Verification items for the finished model (mm, model axes). A direction names the side the tool comes from. Give positions to 0.01 mm unless a question says otherwise; leave off trailing zeros. Answer in a Markdown table with one row per item.
```python
from build123d import *

# Parameters (mm, degrees)
SKETCH1_R           = 13
BOSS_EXTRUDE1_DEPTH = 2
CUT_EXTRUDE1_DEPTH  = 2
CUT_EXTRUDE2_DEPTH  = 2


with BuildPart() as part:
    # Sketch1 → Boss-Extrude1 (new body)
    with BuildSketch(Plane.XY):
        Circle(SKETCH1_R)
    extrude(amount=BOSS_EXTRUDE1_DEPTH)

    # Sketch2 → Cut-Extrude1 (cut)
    with BuildSketch(Plane.XY.offset(2)):
        with BuildLine():
            Line((1.85, 2.101784956), (1.85, -2.101784956))
            ThreePointArc((1.85, -2.101784956), (0, -2.8), (-1.85, -2.101784956))
            Line((-1.85, -2.101784956), (-1.85, 2.101784956))
            ThreePointArc((-1.85, 2.101784956), (0, 2.8), (1.85, 2.101784956))
        make_face()
    extrude(amount=-CUT_EXTRUDE1_DEPTH, mode=Mode.SUBTRACT)

    # Sketch3 → Cut-Extrude2 (cut)
    with BuildSketch(Plane.XY.offset(2)):
        with BuildLine():
            Line((-0.421898485, 5.3), (0.421898485, 5.3))
            Line((0.421898485, 5.3), (1.025755042, 11.638206547))
            add(Edge.make_bspline(
                [(-1.025755042, 11.638206547), (0, 12.476130474), (1.025755042, 11.638206547)],
                knots=[0, 0, 0, 1, 1, 1], degree=2))
            Line((-1.025755042, 11.638206547), (-0.421898485, 5.3))
        make_face()
        with BuildLine():
            Line((2.039039374, 4.910225735), (4.571954624, 10.751616435))
            add(Edge.make_bspline(
                [(2.62085259, 11.385567915), (3.85533634, 11.865505185), (4.571954624, 10.751616435)],
                knots=[0, 0, 0, 1, 1, 1], degree=2))
            Line((2.62085259, 11.385567915), (1.236540767, 5.170973338))
            Line((1.236540767, 5.170973338), (2.039039374, 4.910225735))
        make_face()
        with BuildLine():
            Line((3.456584881, 4.039804363), (7.670619433, 8.812583195))
            add(Edge.make_bspline(
                [(6.01091291, 10.018430567), (7.333285498, 10.093401577), (7.670619433, 8.812583195)],
                knots=[0, 0, 0, 1, 1, 1], degree=2))
            Line((6.01091291, 10.018430567), (2.773938793, 4.535775778))
            Line((2.773938793, 4.535775778), (3.456584881, 4.039804363))
        make_face()
        with BuildLine():
            Line((4.535775778, 2.773938793), (10.018430567, 6.01091291))
            add(Edge.make_bspline(
                [(8.812583195, 7.670619433), (10.093401577, 7.333285498), (10.018430567, 6.01091291)],
                knots=[0, 0, 0, 1, 1, 1], degree=2))
            Line((8.812583195, 7.670619433), (4.039804363, 3.456584881))
            Line((4.039804363, 3.456584881), (4.535775778, 2.773938793))
        make_face()
        with BuildLine():
            Line((5.170973338, 1.236540767), (11.385567915, 2.62085259))
            add(Edge.make_bspline(
                [(10.751616435, 4.571954624), (11.865505185, 3.85533634), (11.385567915, 2.62085259)],
                knots=[0, 0, 0, 1, 1, 1], degree=2))
            Line((10.751616435, 4.571954624), (4.910225735, 2.039039374))
            Line((4.910225735, 2.039039374), (5.170973338, 1.236540767))
        make_face()
        with BuildLine():
            Line((5.3, -0.421898485), (11.638206547, -1.025755042))
            add(Edge.make_bspline(
                [(11.638206547, 1.025755042), (12.476130474, 0), (11.638206547, -1.025755042)],
                knots=[0, 0, 0, 1, 1, 1], degree=2))
            Line((11.638206547, 1.025755042), (5.3, 0.421898485))
            Line((5.3, 0.421898485), (5.3, -0.421898485))
        make_face()
        with BuildLine():
            Line((4.910225735, -2.039039374), (10.751616435, -4.571954624))
            add(Edge.make_bspline(
                [(11.385567915, -2.62085259), (11.865505185, -3.85533634), (10.751616435, -4.571954624)],
                knots=[0, 0, 0, 1, 1, 1], degree=2))
            Line((11.385567915, -2.62085259), (5.170973338, -1.236540767))
            Line((5.170973338, -1.236540767), (4.910225735, -2.039039374))
        make_face()
        with BuildLine():
            Line((4.039804363, -3.456584881), (8.812583195, -7.670619433))
            add(Edge.make_bspline(
                [(10.018430567, -6.01091291), (10.093401577, -7.333285498), (8.812583195, -7.670619433)],
                knots=[0, 0, 0, 1, 1, 1], degree=2))
            Line((10.018430567, -6.01091291), (4.535775778, -2.773938793))
            Line((4.535775778, -2.773938793), (4.039804363, -3.456584881))
        make_face()
        with BuildLine():
            Line((2.773938793, -4.535775778), (6.01091291, -10.018430567))
            add(Edge.make_bspline(
                [(7.670619433, -8.812583195), (7.333285498, -10.093401577), (6.01091291, -10.018430567)],
                knots=[0, 0, 0, 1, 1, 1], degree=2))
            Line((7.670619433, -8.812583195), (3.456584881, -4.039804363))
            Line((3.456584881, -4.039804363), (2.773938793, -4.535775778))
        make_face()
        with BuildLine():
            Line((1.236540767, -5.170973338), (2.62085259, -11.385567915))
            add(Edge.make_bspline(
                [(4.571954624, -10.751616435), (3.85533634, -11.865505185), (2.62085259, -11.385567915)],
                knots=[0, 0, 0, 1, 1, 1], degree=2))
            Line((4.571954624, -10.751616435), (2.039039374, -4.910225735))
            Line((2.039039374, -4.910225735), (1.236540767, -5.170973338))
        make_face()
        with BuildLine():
            Line((-0.421898485, -5.3), (-1.025755042, -11.638206547))
            add(Edge.make_bspline(
                [(1.025755042, -11.638206547), (0, -12.476130474), (-1.025755042, -11.638206547)],
                knots=[0, 0, 0, 1, 1, 1], degree=2))
            Line((1.025755042, -11.638206547), (0.421898485, -5.3))
            Line((0.421898485, -5.3), (-0.421898485, -5.3))
        make_face()
        with BuildLine():
            Line((-2.039039374, -4.910225735), (-4.571954624, -10.751616435))
            add(Edge.make_bspline(
                [(-2.62085259, -11.385567915), (-3.85533634, -11.865505185), (-4.571954624, -10.751616435)],
                knots=[0, 0, 0, 1, 1, 1], degree=2))
            Line((-2.62085259, -11.385567915), (-1.236540767, -5.170973338))
            Line((-1.236540767, -5.170973338), (-2.039039374, -4.910225735))
        make_face()
        with BuildLine():
            Line((-3.456584881, -4.039804363), (-7.670619433, -8.812583195))
            add(Edge.make_bspline(
                [(-6.01091291, -10.018430567), (-7.333285498, -10.093401577), (-7.670619433, -8.812583195)],
                knots=[0, 0, 0, 1, 1, 1], degree=2))
            Line((-6.01091291, -10.018430567), (-2.773938793, -4.535775778))
            Line((-2.773938793, -4.535775778), (-3.456584881, -4.039804363))
        make_face()
        with BuildLine():
            Line((-4.535775778, -2.773938793), (-10.018430567, -6.01091291))
            add(Edge.make_bspline(
                [(-8.812583195, -7.670619433), (-10.093401577, -7.333285498), (-10.018430567, -6.01091291)],
                knots=[0, 0, 0, 1, 1, 1], degree=2))
            Line((-8.812583195, -7.670619433), (-4.039804363, -3.456584881))
            Line((-4.039804363, -3.456584881), (-4.535775778, -2.773938793))
        make_face()
        with BuildLine():
            Line((-5.170973338, -1.236540767), (-11.385567915, -2.62085259))
            add(Edge.make_bspline(
                [(-10.751616435, -4.571954624), (-11.865505185, -3.85533634), (-11.385567915, -2.62085259)],
                knots=[0, 0, 0, 1, 1, 1], degree=2))
            Line((-10.751616435, -4.571954624), (-4.910225735, -2.039039374))
            Line((-4.910225735, -2.039039374), (-5.170973338, -1.236540767))
        make_face()
        with BuildLine():
            Line((-5.3, 0.421898485), (-11.638206547, 1.025755042))
            add(Edge.make_bspline(
                [(-11.638206547, -1.025755042), (-12.476130474, 0), (-11.638206547, 1.025755042)],
                knots=[0, 0, 0, 1, 1, 1], degree=2))
            Line((-11.638206547, -1.025755042), (-5.3, -0.421898485))
            Line((-5.3, -0.421898485), (-5.3, 0.421898485))
        make_face()
        with BuildLine():
            Line((-4.910225735, 2.039039374), (-10.751616435, 4.571954624))
            add(Edge.make_bspline(
                [(-11.385567915, 2.62085259), (-11.865505185, 3.85533634), (-10.751616435, 4.571954624)],
                knots=[0, 0, 0, 1, 1, 1], degree=2))
            Line((-11.385567915, 2.62085259), (-5.170973338, 1.236540767))
            Line((-5.170973338, 1.236540767), (-4.910225735, 2.039039374))
        make_face()
        with BuildLine():
            Line((-4.039804363, 3.456584881), (-8.812583195, 7.670619433))
            add(Edge.make_bspline(
                [(-10.018430567, 6.01091291), (-10.093401577, 7.333285498), (-8.812583195, 7.670619433)],
                knots=[0, 0, 0, 1, 1, 1], degree=2))
            Line((-10.018430567, 6.01091291), (-4.535775778, 2.773938793))
            Line((-4.535775778, 2.773938793), (-4.039804363, 3.456584881))
        make_face()
        with BuildLine():
            Line((-2.773938793, 4.535775778), (-6.01091291, 10.018430567))
            add(Edge.make_bspline(
                [(-7.670619433, 8.812583195), (-7.333285498, 10.093401577), (-6.01091291, 10.018430567)],
                knots=[0, 0, 0, 1, 1, 1], degree=2))
            Line((-7.670619433, 8.812583195), (-3.456584881, 4.039804363))
            Line((-3.456584881, 4.039804363), (-2.773938793, 4.535775778))
        make_face()
        with BuildLine():
            Line((-1.236540767, 5.170973338), (-2.62085259, 11.385567915))
            add(Edge.make_bspline(
                [(-4.571954624, 10.751616435), (-3.85533634, 11.865505185), (-2.62085259, 11.385567915)],
                knots=[0, 0, 0, 1, 1, 1], degree=2))
            Line((-4.571954624, 10.751616435), (-2.039039374, 4.910225735))
            Line((-2.039039374, 4.910225735), (-1.236540767, 5.170973338))
        make_face()
    extrude(amount=-CUT_EXTRUDE2_DEPTH, mode=Mode.SUBTRACT)


solid = part.part
```
Item 1: Tool access check on faces 3 (the flat face through (0.72, 8.42, 1.01)), 4 (the flat face through (0, 3, 0)). Record the directions out of +Z, -Z, +X, -X, +Y, -Y that give a thin tool (end or side, any length) a straight path to the whole face; none if there is none.
Reported:
| item | result |
|---|---|
| face 3 | +Z, -Z |
| face 4 | -Z, +X, -X, +Y, -Y |
Item 2: Go/stop test with flat-tipped pins: pin 1 (2 mm diameter, centred on x = 3, y = -2.5, fed in from -Z); pin 2 (0.6 mm diameter, centred on y = 1, z = 1.5, fed in from +X); pin 3 (1 mm diameter, centred on y = 1, z = 1, fed in from -X). Record where each tip stops, or that it passes through.
Reported:
| item | result |
|---|---|
| pin 1 | stops at z = 0 |
| pin 2 | stops at x = 12.98 |
| pin 3 | stops at x = -12.99 |
Item 3: Sectioned sample at A-A (y = 0). State how many separate pieces and enclosed holes the cut face has, and give its area (3 significant figures).
Reported:
| item | result |
|---|---|
| separate pieces | 4 |
| enclosed holes | 0 |
| area | 17.6 mm^2 |
Item 4: Release check for a two-part mould opening along Y. For faces 1 (the flat face through (0, 3, 2)), 2 (the flat face through (1.919, -8.235, 1.014)) record: released by +Y, released by -Y, zero draft, split by the parting line, or undercut.
Reported:
| item | result |
|---|---|
| face 1 | zero draft |
| face 2 | undercut |
Item 5: Scan lines: L1, parallel to Y at x = 8, z = 1.5; L2, parallel to X at y = 4.75, z = 1.15; L3, parallel to Y at x = 3, z = 0.95. Record each from-to range of solid material in increasing order. Write a range as [from, to].
Reported:
| item | result |
|---|---|
| L1 | y = [-10.25, -6.95], [-4.82, -3.38], [-1.87, -0.68], [0.68, 1.87], [3.38, 4.82], [6.95, 10.25] |
| L2 | x = [-12.1, -7.88], [-5.5, -4.08], [-2.9, 2.9], [4.08, 5.5], [7.88, 12.1] |
| L3 | y = [-12.65, -11.5], [-7.13, -4.92], [-4.37, 4.37], [4.92, 7.13], [11.5, 12.65] |
